Can you work these out from the model? Positions are in its coordinate system, mm. A direction names the side the tool comes from. Give positions to 0.01 mm unless a question says otherwise; leave off trailing zeros. Loops run counter-clockwise (first coordinate to the right, second up) from the corner with the lowest first, then second, coordinate; pieces in that order, holes last. Notation, with made-up numbers: M 14,45.5 L 55,45.5 A26 cw 55,78.5 Z; hole C 38.5,-34.75 d11. An arc over 180 degrees is marked long. Use CSV: the item, a comma, the result in double quotes.
Autodesk Inventor part; units mm, degrees
ref_plane "YZ Plane" through (0, 0, 0) normal (1, 0, 0) x (0, 1, 0)
ref_plane "XZ Plane" through (0, 0, 0) normal (0, 1, 0) x (-1, 0, 0)
ref_plane "XY Plane" through (0, 0, 0) normal (0, 0, 1) x (1, 0, 0)
sketch "Sketch1" plane through (0, 0, 0) normal (0, 1, 0) x (-1, 0, 0)
  line L0 (0, 0) -> (0, -233.234) construction
  line L1 (-3, 0) -> (-3, -233.234)
  line L2 (3, -233.234) -> (3, 0)
  arc A0 (3, 0) -> (-3, 0) centre (0, 0) ccw
  arc A1 (-3, -233.234) -> (3, -233.234) centre (0, -233.234) ccw
  circle A2 centre (0, 0) radius 1.5
  circle A3 centre (0, -233.234) radius 1.5
  circle A4 centre (0, -103.234) radius 1.5
  arc A5 (3, -106.234) -> (3, -230.234) centre (599.7881, -168.234) ccw
  arc A6 (-3, -106.234) -> (-3, -230.234) centre (593.7881, -168.234) ccw
  point P0 (0, -116.617)
  dimension "d0" = 6
  dimension "d1" = 233.234
  dimension "d2" = 3
  dimension "d3" = 3
  dimension "d16" = 3
  dimension "d17" = 103.234
  dimension "d20" = 600
  dimension "d21" = 3
  dimension "d22" = 3
  dimension "d23" = 600
extrude "Extrusion1" add sketch "Sketch1" along normal blind 10 contours A0 L2 A5 A1 L1 | L1 A6
Q1. I want a section at B-B, the plane z = -63.5. Please give me the cut outline in (x, y).
Model answer:
outline,"M -3,0 L 3,0 L 3,10 L -3,10 Z"
Q2. Please list where these lines run through material, in increasing order: L1, parallel to Z at x = 0.5, y = 0.5; L2, parallel to Z at x = 1.25, y = 0.5; L3, parallel to X at y = 4.75, z = -82. Write a range as from..to.
Model answer:
L1,"-236.19..-234.65, -231.82..-104.65, -101.82..-1.41, 1.41..2.96"
L2,"-235.96..-234.06, -232.4..-104.06, -102.4..-0.83, 0.83..2.73"
L3,"-3..3"
Q3. I'm going to push flat-ended pins straight in: P1, Ø3, axis at x = 3, y = 5.5, coming from the -Z side; P2, Ø2.5, axis at y = 4, z = -232, coming from the +X side; P3, Ø2, axis at x = 1.5, y = 6, coming from the -Z side. Where does each tip first touch, or does it pass through?
Model answer:
P1,"z = -235.83"
P2,"x = 3"
P3,"z = -236.19"
Q4. For faces 1 (the cylindrical face through (6.21, 4.93, -169.1)), 2 (the flat face through (3, 5, -52)), which set-ups out of +Z, -Z, +X, -X, +Y, -Y let a thin tool reach every point of the face, with its end or its side?
Model answer:
face 1,"+X, +Y, -Y"
face 2,"+Z, +X, +Y, -Y"
Q5. If we mould it in two halves opening along Z, with no side actions, what happens to faces 3 (the cylindrical face through (-0.066, 4.93, -236.233)), 4 (the cylindrical face through (0.21, 4.93, -169.1)), 5 (the flat face through (2, 10, -115))? For each: released by +Z, released by -Z, zero draft, split by the parting line, or undercut.
Model answer:
face 3,"released by -Z"
face 4,"undercut"
face 5,"zero draft"
Q6. I want a section at A-A, the plane y = 3.5. Please give me the cut outline in (x, z).
Model answer:
outline,"M -3,-233.23 A3 ccw 3,-233.23 L 3,-230.23 A600 ccw 3,-106.23 L 3,0 A3 ccw -3,0 L -3,-106.23 A600 cw -3,-230.23 Z; hole C 0,-233.23 d3; hole C 0,-103.23 d3; hole C 0,0 d3"
